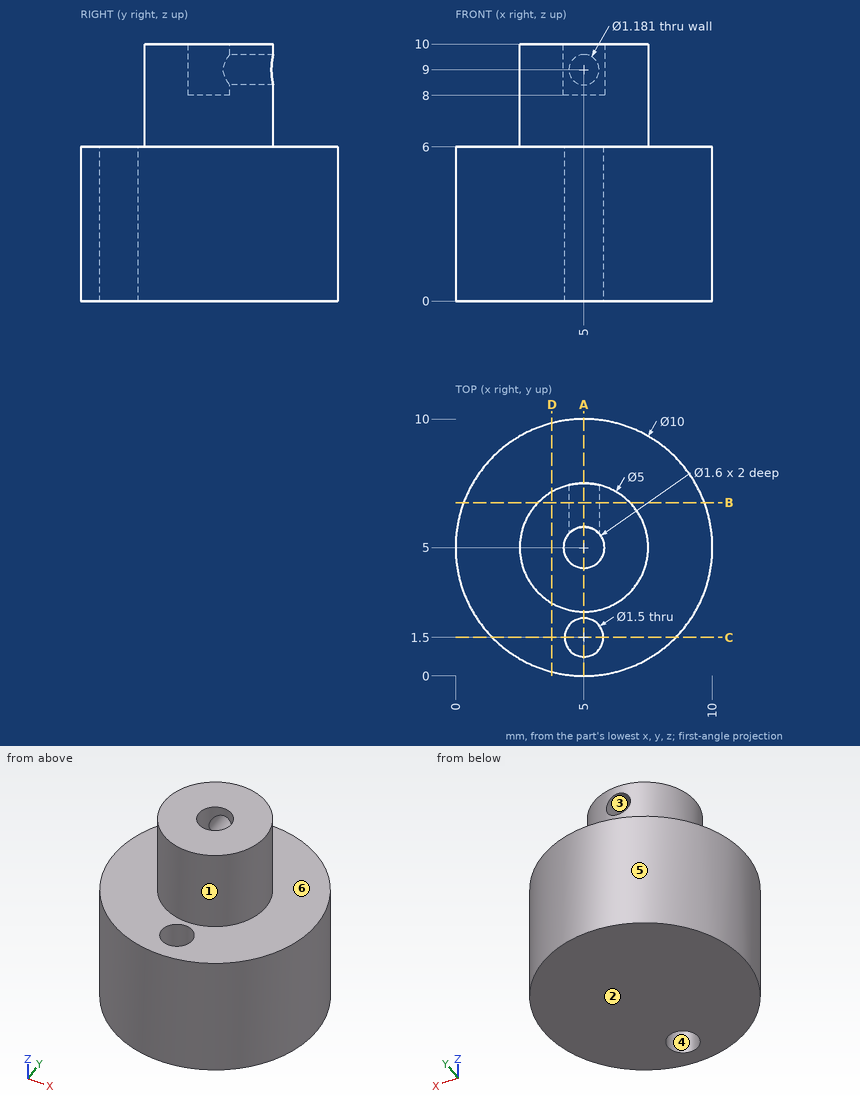
Can you work these out from the drawing? Everything is in mm from the part's minimum corner. A direction names the side the tool comes from. Give positions to 0.01 mm unless a question says otherwise; leave off trailing zeros. Order: outer loops, then holes, each group sorted by start corner. A loop starts at its lowest first (then second) coordinate and runs counter-clockwise, first axis right, second up. Notation, with made-up numbers: M 1,8.25 L 58,8.25 A24 ccw 58,19.25 Z; hole C 13.25,62 d9. An arc over 180 degrees is marked long. One line per question, with ' | ' between items.
1. I'm going to push flat-ended pins straight in: pin 1 (1.1 mm diameter, centred on x = 5, z = 9, fed in from -Y); pin 2 (4 mm diameter, centred on x = 8, z = 6.5, fed in from +Y); pin 3 (2 mm diameter, centred on y = 6, z = 8.5, fed in from -X). Where does each tip first touch, or does it pass through?
Results:
pin 1: y = 2.5 | pin 2: y = 9.89 | pin 3: x = 2.5
2. I want a section at C-C (y = 1.5). List the corners of the cut face in (x, z) for me, and give its area (3 significant figures).
Results:
outline: M 1.43,0 L 4.25,0 L 4.25,6 L 1.43,6 Z; M 5.75,0 L 8.57,0 L 8.57,6 L 5.75,6 Z | area: 33.8 mm²
3. We'd pull the mould along X, two halves only. Please class the marked faces 1, 2, 3 and 4: +X half, -X half, draft (parallel to the pull), parting line (faces both ways), or undercut.
Results:
face 1: parting line | face 2: draft | face 3: undercut | face 4: undercut
4. If I drill on line 1 (Y direction, x = 5, z = 1.95); line 2 (Y direction, x = 4.5, z = 1.75); line 3 (Y direction, x = 5, z = 8.6), over which ranges is the centre line in solid material (lowest first)?
Results:
line 1: 0 to 0.75, 2.25 to 10 | line 2: 0.03 to 0.94, 2.06 to 9.97 | line 3: 2.5 to 4.2
5. I want a section at D-D (x = 3.75). List the corners of the cut face in (y, z) for me.
Results:
outline: M 0.16,0 L 9.84,0 L 9.84,6 L 7.17,6 L 7.17,10 L 2.83,10 L 2.83,6 L 0.16,6 Z
6. For the marked faces 5 and 6, which set-ups out of +Z, -Z, +X, -X, +Y, -Y let a thin tool reach every point of the face, with its end or its side?
Results:
face 5: +Z, -Z | face 6: +Z
7. I want a section at A-A (x = 5). List the corners of the cut face in (y, z) for me.
Results:
outline: M 0,0 L 0.75,0 L 0.75,6 L 0,6 Z; M 2.25,0 L 10,0 L 10,6 L 7.5,6 L 7.5,8.41 L 5.8,8.41 L 5.8,8 L 4.2,8 L 4.2,10 L 2.5,10 L 2.5,6 L 2.25,6 Z; M 5.8,9.59 L 7.5,9.59 L 7.5,10 L 5.8,10 Z
8. I want a section at B-B (y = 6.75). List the corners of the cut face in (x, z) for me.
Results:
outline: M 0.32,0 L 9.68,0 L 9.68,6 L 6.79,6 L 6.79,10 L 3.21,10 L 3.21,6 L 0.32,6 Z; hole C 5,9 d1.18
